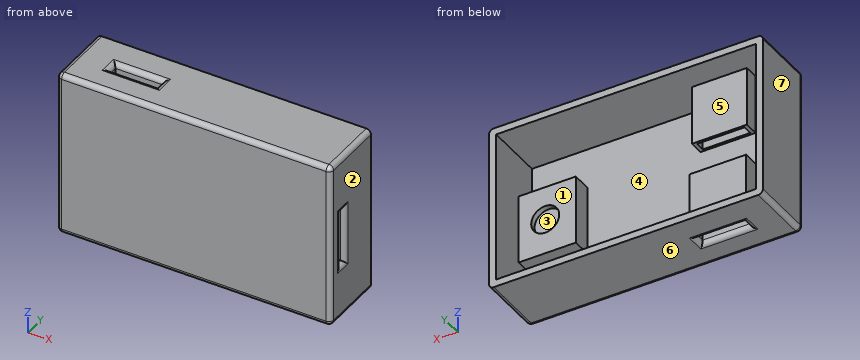
```python
from build123d import *

# Parameters (mm, degrees)
SKETCH1_W           = 115
SKETCH1_H           = 70
BOSS_EXTRUDE1_DEPTH = 28
SHELL2_T            = -3
SKETCH2_W           = 20
SKETCH2_H           = 4
CUT_EXTRUDE1_DEPTH  = 95.816928868
SKETCH4_W           = 23.796796
SKETCH4_H           = 8.165514589
SKETCH4_W_2         = 20
SKETCH4_H_2         = 4
BOSS_EXTRUDE2_DEPTH = 25
SKETCH5_W           = 23.125103044
SKETCH5_H           = 6.017817829
SKETCH5_W_2         = 20
SKETCH5_H_2         = 4
BOSS_EXTRUDE3_DEPTH = 25
FILLET2_R           = 2
FILLET3_R           = 2
SKETCH9_W           = 29.136235749
SKETCH9_H           = 7.961178331
BOSS_EXTRUDE4_DEPTH = 25
SKETCH11_W          = 23.614359243
SKETCH11_H          = 3.227216001
CUT_EXTRUDE4_DEPTH  = 101.543522914
FILLET4_R           = 2
CUT_EXTRUDE5_REACH  = 71.124
SKETCH12_R          = 5.884599132
SKETCH13_W          = 29.136235749
SKETCH13_H          = 7.961178331
BOSS_EXTRUDE5_DEPTH = 2


with BuildPart() as part:
    # Sketch1 → Boss-Extrude1 (new body)
    with BuildSketch(Plane(origin=(0, 0, 0), x_dir=(1, 0, 0), z_dir=(0, 1, 0))):
        Rectangle(SKETCH1_W, SKETCH1_H)
    extrude(amount=BOSS_EXTRUDE1_DEPTH)

    # Shell2
    shell2_openings = [part.faces().sort_by_distance(p)[0] for p in [
        (0, 28, 0),
    ]]
    offset(amount=SHELL2_T, openings=shell2_openings, kind=Kind.INTERSECTION)

    # Sketch2 → Cut-Extrude1 (cut, through all)
    with BuildSketch(Plane.XY.offset(35)):
        with Locations((-32.5, 13.8542792)):
            Rectangle(SKETCH2_W, SKETCH2_H)
    extrude(amount=-CUT_EXTRUDE1_DEPTH, mode=Mode.SUBTRACT)

    # Sketch4 → Boss-Extrude2 (add)
    with BuildSketch(Plane.XY.offset(-32)):
        with Locations((-32.5, 13.854279201)):
            Rectangle(SKETCH4_W, SKETCH4_H)
        with Locations((-32.5, 13.8542792)):
            Rectangle(SKETCH4_W_2, SKETCH4_H_2, mode=Mode.SUBTRACT)
    extrude(amount=BOSS_EXTRUDE2_DEPTH)

    # Sketch5 → Boss-Extrude3 (add)
    with BuildSketch(Plane(origin=(0, 0, 32), x_dir=(-1, 0, 0), z_dir=(0, 0, -1))):
        with Locations((32.5, 13.854279201)):
            Rectangle(SKETCH5_W, SKETCH5_H)
        with Locations((32.5, 13.8542792)):
            Rectangle(SKETCH5_W_2, SKETCH5_H_2, mode=Mode.SUBTRACT)
    extrude(amount=BOSS_EXTRUDE3_DEPTH)

    # Fillet2
    fillet2_edges = [part.edges().sort_by_distance(p)[0] for p in [
        (0, 0, 35),
        (-57.5, 0, 0),
        (0, 0, -35),
        (57.5, 0, 0),
        (57.5, 14, 35),
        (-57.5, 14, 35),
        (-57.5, 14, -35),
        (57.5, 14, -35),
    ]]
    fillet(fillet2_edges, radius=FILLET2_R)

    # Fillet3
    fillet3_edges = [part.edges().sort_by_distance(p)[0] for p in [
        (-42.5, 13.8542792, -35),
        (-32.5, 15.8542792, -35),
        (-22.5, 13.8542792, -35),
        (-32.5, 11.8542792, -35),
        (-42.5, 13.8542792, 35),
        (-32.5, 11.8542792, 35),
        (-22.5, 13.8542792, 35),
        (-32.5, 15.8542792, 35),
    ]]
    fillet(fillet3_edges, radius=FILLET3_R)

    # Sketch9 → Boss-Extrude4 (add)
    with BuildSketch(Plane.ZY.offset(-57.5)):
        with Locations((-0.368841187, 8.308427345)):
            Rectangle(SKETCH9_W, SKETCH9_H)
    extrude(amount=BOSS_EXTRUDE4_DEPTH)

    # Sketch11 → Cut-Extrude4 (cut, through all)
    with BuildSketch(Plane.ZY.offset(-32.5)):
        with Locations((-0.368841187, 8.308427345)):
            Rectangle(SKETCH11_W, SKETCH11_H)
    extrude(amount=-CUT_EXTRUDE4_DEPTH, mode=Mode.SUBTRACT)

    # Fillet4
    fillet4_edges = [part.edges().sort_by_distance(p)[0] for p in [
        (57.5, 8.308427345, 11.438338435),
        (57.5, 6.694819344, -0.368841187),
        (57.5, 8.308427345, -12.176020808),
        (57.5, 9.922035345, -0.368841187),
    ]]
    fillet(fillet4_edges, radius=FILLET4_R)

    # Sketch12 → Cut-Extrude5 (cut, up to next)
    with BuildSketch(Plane(origin=(0, 12.28901651, 0), x_dir=(1, 0, 0), z_dir=(0, 1, 0)), mode=Mode.PRIVATE) as cut_extrude5_sk1:
        with Locations(Location((43.35506163, 0, 0), (0, 0, 270))):
            Circle(SKETCH12_R)
    cut_extrude5_tool1 = extrude(cut_extrude5_sk1.sketch, amount=-CUT_EXTRUDE5_REACH, mode=Mode.PRIVATE) & part.part
    add(cut_extrude5_tool1.solids().sort_by_distance((43.355062, 12.289017, 0))[0], mode=Mode.SUBTRACT)

    # Sketch13 → Boss-Extrude5 (add)
    with BuildSketch(Plane.ZY.offset(-32.5)):
        with Locations((-0.368841187, 8.308427345)):
            Rectangle(SKETCH13_W, SKETCH13_H)
    extrude(amount=BOSS_EXTRUDE5_DEPTH)


solid = part.part
```
Work out the finished part from the listing and answer in its coordinate system (mm). Face numbers are marked on the shaded views. A direction names the side the tool comes from. Round coordinates to 2 decimals unless told otherwise and drop trailing zeros. Loops run counter-clockwise (first coordinate to the right, second up) from the corner with the lowest first, then second, coordinate; pieces in that order, holes last. Notation, with made-up numbers: M 69.5,-22.5 L 125.5,-22.5 A25 ccw 125.5,12.5 Z; hole C -38.75,-32.5 d6. An arc over 180 degrees is marked long. One line per question, with ' | ' between items.
Q1. A tool of negligible diameter and unlimited length cuts with its end or side. For the marked faces 1, 2, 3 and 4, from which of +Z, -Z, +X, -X, +Y, -Y can it reach the whole face along a straight path? Write none if from no direction.
Conclusion:
face 1: +Y | face 2: +Z, -Z, +X, +Y, -Y | face 3: +X | face 4: none
Q2. Find section D-D, the plane x = -9. Give the vertices of the cut face in (y, z).
Conclusion:
outline: M 0,-33 A2 ccw 2,-35 L 28,-35 L 28,-32 L 3,-32 L 3,32 L 28,32 L 28,35 L 2,35 A2 ccw 0,33 Z
Q3. Each of these flat-tipped pins is pushed along its axis until it touches: pin 1 Ø2.5 at (y, z) = (8.5, 3) entering from +X; pin 2 Ø22 at (x, z) = (-34, -17) entering from +Y; pin 3 Ø6 at (x, z) = (3, 18.5) entering from +Y. Where does it stop, or does it pass through?
Conclusion:
pin 1: stops at x = 32.5 | pin 2: stops at y = 17.94 | pin 3: stops at y = 3
Q4. Find section A-A, the plane z = -29. Give the vertices of the cut face in (x, y).
Conclusion:
outline: M -57.5,2 A2 ccw -55.5,0 L 55.5,0 A2 ccw 57.5,2 L 57.5,28 L 54.5,28 L 54.5,3 L -54.5,3 L -54.5,28 L -57.5,28 Z; M -44.4,9.77 L -20.6,9.77 L -20.6,17.94 L -44.4,17.94 Z; hole M -42.5,11.85 L -22.5,11.85 L -22.5,15.85 L -42.5,15.85 Z
Q5. Consider line 1 along Z through (x, y) = (37, 9.75); line 2 along Y through (x, z) = (-27, -30); line 3 along Y through (x, z) = (-23, 14). Determine where each line is inside the solid, lowest interval first. Write a range as from..to.
Conclusion:
line 1: z = -35..-32, -14.94..-12.18, 11.44..14.2, 32..35 | line 2: y = 0..3, 9.77..11.85, 15.85..17.94 | line 3: y = 0..3, 10.85..11.85, 15.85..16.86
Q6. Find section C-C, the plane z = 0. Give the vertices of the cut face in (x, y), then the cut area to 3 significant figures.
Conclusion:
outline: M -57.5,2 A2 ccw -55.5,0 L 55.5,0 A2 ccw 57.5,2 L 57.5,4.69 A2 ccw 55.5,6.69 L 32.5,6.69 L 32.5,9.92 L 37.47,9.92 L 37.47,12.29 L 30.5,12.29 L 30.5,4.33 L 54.5,4.33 L 54.5,3 L -54.5,3 L -54.5,28 L -57.5,28 Z; M 49.24,9.92 L 55.5,9.92 A2 ccw 57.5,11.92 L 57.5,28 L 54.5,28 L 54.5,12.29 L 49.24,12.29 Z | area: 574 mm2
Q7. The mould has two halves that part along X. Classify the marked faces 5, 6 and 7: +X half, -X half, draft (parallel to the pull), parting line (faces both ways), or undercut.
Conclusion:
face 5: undercut | face 6: draft | face 7: -X half
